Source: CAD feature listing. Evaluate the final solid. Frame: model axes, mm. A direction names the side the tool comes from. Give positions to 0.01 mm unless a question says otherwise; leave off trailing zeros.
from build123d import *

# Parameters (mm, degrees)
SKETCH2_R           = 39.5
BOSS_EXTRUDE1_DEPTH = 1
SKETCH4_R           = 41
BOSS_EXTRUDE2_DEPTH = 1
SKETCH5_R           = 42
BOSS_EXTRUDE3_DEPTH = 7
SKETCH6_R           = 35
BOSS_EXTRUDE4_DEPTH = 3
BOSS_EXTRUDE5_DEPTH = 1
CIRPATTERN1_COUNT   = 16
SKETCH8_W           = 20
SKETCH8_H           = 40
BOSS_EXTRUDE6_DEPTH = 42
SKETCH9_R           = 20
BOSS_EXTRUDE7_DEPTH = 20
SKETCH10_R          = 10
BOSS_EXTRUDE8_DEPTH = 10
SKETCH11_R          = 10
BOSS_EXTRUDE9_DEPTH = 10


with BuildPart() as part:
    # Sketch1 → Revolve1 (revolve)
    with BuildSketch(Plane(origin=(0, 0, 0), x_dir=(0, 0, -1), z_dir=(1, 0, 0)), mode=Mode.PRIVATE) as revolve1_sk:
        with BuildLine():
            Line((0, 0), (-42, 0))
            ThreePointArc((-42, 0), (-39.032396198, 11.288859787), (-31.263157895, 20))
            Line((-31.263157895, 20), (0, 20))
            Line((0, 20), (0, 0))
        make_face()
    revolve(revolve1_sk.sketch.rotate(Axis((0, 0, 0), (0, 1, 0)), 180), axis=Axis((0, 0, 0), (0, 1, 0)))

    # Sketch2 → Boss-Extrude1 (add)
    with BuildSketch(Plane.XZ):
        with Locations(Location((0, 0, 0), (0, 0, 270))):
            Circle(SKETCH2_R)
    extrude(amount=BOSS_EXTRUDE1_DEPTH)

    # Sketch3 → Revolve2 (revolve)
    with BuildSketch(Plane.XY, mode=Mode.PRIVATE) as revolve2_sk:
        with BuildLine():
            Line((0, -1), (0, -21))
            Line((0, -21), (-40, -21))
            ThreePointArc((-40, -21), (-41.376973739, -11), (-40, -1))
            Line((-40, -1), (0, -1))
        make_face()
    revolve(revolve2_sk.sketch.rotate(Axis((0, -1, 0), (0, -1, 0)), 90), axis=Axis((0, -1, 0), (0, -1, 0)))

    # Sketch4 → Boss-Extrude2 (add)
    with BuildSketch(Plane.XZ.offset(21)):
        Circle(SKETCH4_R)
    extrude(amount=BOSS_EXTRUDE2_DEPTH)

    # Sketch5 → Boss-Extrude3 (add)
    with BuildSketch(Plane.XZ.offset(22)):
        Circle(SKETCH5_R)
    extrude(amount=BOSS_EXTRUDE3_DEPTH)

    # Sketch6 → Boss-Extrude4 (add)
    with BuildSketch(Plane.XZ.offset(29)):
        Circle(SKETCH6_R)
    extrude(amount=BOSS_EXTRUDE4_DEPTH)

    # Sketch7 → Boss-Extrude5 (add)
    with BuildSketch(Plane.XZ.offset(29)):
        with BuildLine():
            ThreePointArc((37, 0), (38.5, 1.5), (40, 0))
            Line((40, 0), (40.75, 0))
            ThreePointArc((40.75, 0), (38.5, 2.25), (36.25, 0))
            Line((36.25, 0), (37, 0))
        make_face()
        with BuildLine():
            Line((40.75, 0), (40, 0))
            ThreePointArc((40, 0), (38.5, -1.5), (37, 0))
            Line((37, 0), (36.25, 0))
            ThreePointArc((36.25, 0), (38.5, -2.25), (40.75, 0))
        make_face()
    boss_extrude5 = extrude(amount=BOSS_EXTRUDE5_DEPTH)

    # CirPattern1: Boss-Extrude5 ×16 about axis
    cirpattern1_axis = Axis((0, 0, 0), (0, 1, 0))
    for i in range(1, CIRPATTERN1_COUNT):
        add(boss_extrude5.rotate(cirpattern1_axis, i * 360 / CIRPATTERN1_COUNT))

    # Sketch8 → Boss-Extrude6 (add)
    with BuildSketch(Plane(origin=(0, 20, 0), x_dir=(1, 0, 0), z_dir=(0, 1, 0))):
        Rectangle(SKETCH8_W, SKETCH8_H)
    extrude(amount=BOSS_EXTRUDE6_DEPTH)

    # Sketch9 → Boss-Extrude7 (add)
    with BuildSketch(Plane(origin=(10, 0, 0), x_dir=(0, 0, -1), z_dir=(1, 0, 0))):
        with Locations((0, 62)):
            Circle(SKETCH9_R)
    extrude(amount=-BOSS_EXTRUDE7_DEPTH)

    # Sketch10 → Boss-Extrude8 (add)
    with BuildSketch(Plane.ZY.offset(10)):
        with Locations(Location((0, 62, 0), (0, 0, 180))):
            Circle(SKETCH10_R)
    extrude(amount=BOSS_EXTRUDE8_DEPTH)

    # Sketch11 → Boss-Extrude9 (add)
    with BuildSketch(Plane.XZ.offset(32)):
        Circle(SKETCH11_R)
    extrude(amount=BOSS_EXTRUDE9_DEPTH)


solid = part.part
(1) Pin query (flat end, axial travel): pin 1 Ø2 at (y, z) = (-8, -7.5) entering from +X; pin 2 Ø10 at (y, z) = (-21.5, -16) entering from +X; pin 3 Ø2.5 at (x, z) = (-38.5, 0) entering from -Y. Return the tip coordinate at first contact, or that it passes through.
(2) Access query for faces 1 (the flat face through (-29, -30, -27)), 2 (the cylindrical face through (-35.83, -29.49, 16.21)), 3 (the flat face through (37, -30, -16)). Directions: +Z, -Z, +X, -X, +Y, -Y. A direction counts if a zero-diameter tool reaches every point of the face in a straight line with its end or side. Return the directions, or none.
(3) Line query: line 1 along Y through (x, z) = (-12.5, -24.5); line 2 along X through (y, z) = (-26, 0.5); line 3 along X through (y, z) = (74, 5). Output: solid intervals per line, ascending.
(4) Draft query along Y for faces 4 (the cylindrical face through (36.719, -29.493, -15.697)), 5 (the flat face through (-10, 44, 0)), 6 (the flat face through (-25, -29, -25)). Return one class per face: +Y half, -Y half, draft (parallel to the pull), parting line (faces both ways), or undercut.
Checks:
1. pin 1: stops at x = 40.76
1. pin 2: stops at x = 40.53
1. pin 3: stops at y = -29
2. face 1: -Z, -X, -Y
2. face 2: -Y
2. face 3: -Z, +X, -Y
3. line 1: y = -32 to 20
3. line 2: x = -42 to 42
3. line 3: x = -10 to 10
4. face 4: draft
4. face 5: undercut
4. face 6: -Y half
